Autodesk Inventor part; units mm, degrees
ref_plane "YZ Plane" through (0, 0, 0) normal (1, 0, 0) x (0, 1, 0)
ref_plane "XZ Plane" through (0, 0, 0) normal (0, 1, 0) x (-1, 0, 0)
ref_plane "XY Plane" through (0, 0, 0) normal (0, 0, 1) x (1, 0, 0)
sketch "Эскиз1" plane through (0, 0, 0) normal (0, 0, 1) x (1, 0, 0)
  arc A0 (-17.4305, 17.6734) -> (-22.4305, 12.6734) centre (-17.4305, 12.6734) ccw
  line L0 (-22.4305, 12.6734) -> (-22.4305, -4.8714)
  arc A1 (-22.4305, -4.8714) -> (-17.4305, -9.8714) centre (-17.4305, -4.8714) ccw
  line L1 (-17.4305, -9.8714) -> (-4.1609, -9.8714)
  line L2 (-4.1609, -9.8714) -> (-4.1609, -17.7214)
  arc A2 (-4.1609, -17.7214) -> (-0.1609, -21.7214) centre (-0.1609, -17.7214) ccw
  line L3 (-0.1609, -21.7214) -> (9.8391, -21.7214)
  arc A3 (9.8391, -21.7214) -> (14.8391, -16.7214) centre (9.8391, -16.7214) ccw
  line L4 (14.8391, -16.7214) -> (14.8391, -9.8714)
  line L5 (19.8391, -9.8714) -> (19.8391, 12.6734)
  arc A4 (19.8391, 12.6734) -> (14.8391, 17.6734) centre (14.8391, 12.6734) ccw
  line L6 (14.8391, 17.6734) -> (-17.4305, 17.6734)
  circle A5 centre (-11.2957, 3.901) radius 2.5
  circle A6 centre (4.8391, -17.7214) radius 1.5
  line L7 (14.8391, -9.8714) -> (19.8391, -9.8714)
  circle A7 centre (-11.2957, 13.465) radius 0.75
  circle A8 centre (-11.2957, -5.8075) radius 0.75
  point P0 (0, 0)
  dimension "d0" = 5
extrude "Выдавливание1" add sketch "Эскиз1" along normal blind 2
chamfer "Фаска3" distance 2 angle 45 1 edges at (-12.0457, -5.8075, 0)
chamfer "Фаска4" distance 2 angle 45 1 edges at (-12.0457, 13.465, 0)
properties part number "Верт держатели-2 правый"
Here's how the part is built. I have some questions about the finished solid (model axes, mm). A direction names the side the tool comes from. Give positions to 0.01 mm unless a question says otherwise; leave off trailing zeros. Order: outer loops, then holes, each group sorted by start corner. A loop starts at its lowest first (then second) coordinate and runs counter-clockwise, first axis right, second up. Notation, with made-up numbers: M 57.25,83 L 106.25,83 A11 ccw 106.25,92 Z; hole C -22.5,-4.75 d3. An arc over 180 degrees is marked long. Use a Markdown table: item, result. Add a question column.
1. On a 3-axis mill with a long thin cutter (end or side, diameter ignored), from which of +Z, -Z, +X, -X, +Y, -Y can I reach the whole of each face in a straight line? I mean faces 4 (the flat face through (-1, 17.673, 1)), 5 (the flat face through (-11, -9.871, 1)). Say none if no direction works.
2. Suppose I cut it at B-B (x = -15). List the corners of the cut face in (y, z) for me.
3. For pin 1 Ø1.7 at (x, y) = (-11.3, -5.81) entering from -Z; pin 2 Ø1 at (x, z) = (16.5, 1) entering from -Y; pin 3 Ø0.6 at (y, z) = (-13.5, 0.5) entering from +X, each with a flat end and sliding along its axis, tell me the tip position at first contact or that it passes through.
4. Suppose I cut it at A-A (z = 0.65). List the corners of the cut face in (x, y) for me (1 decimal), and give its area (3 significant figures).
5. Suppose I cut it at C-C (y = -14). List the corners of the cut face in (x, z) for me.
6. If we mould it in two halves opening along X, with no side actions, what happens to faces 1 (the flat face through (-22.43, 4, 1)), 2 (the cylindrical face through (18.336, 16.248, 0.986)), 3 (the cylindrical face through (-13.793, 3.791, 0.986))? For each: +X half, -X half, draft (parallel to the pull), parting line (faces both ways), or undercut.
7. I need wall thicknesses on probe 1 along Y at (x, z) = (5, 1.1); probe 2 along X at (y, z) = (-12.5, 1.7); probe 3 along Y at (x, z) = (-16.5, 0.45). Which ranges of each line are inside material? Lowest first, please. Write a range as from..to.
Results list:
| question | item | result |
|---|---|---|
| 1 | face 4 | +Z, -Z, +X, -X, +Y |
| 1 | face 5 | +Z, -Z, -X, -Y |
| 2 | outline | M -9.87,0 L 17.67,0 L 17.67,2 L -9.87,2 Z |
| 3 | pin 1 | stops at z = 1.89 |
| 3 | pin 2 | stops at y = -9.87 |
| 3 | pin 3 | stops at x = 14.84 |
| 4 | outline | M -22.4,-4.9 A5 ccw -17.4,-9.9 L -4.2,-9.9 L -4.2,-17.7 A4 ccw -0.2,-21.7 L 9.8,-21.7 A5 ccw 14.8,-16.7 L 14.8,-9.9 L 19.8,-9.9 L 19.8,12.7 A5 ccw 14.8,17.7 L -17.4,17.7 A5 ccw -22.4,12.7 Z; hole C -11.3,3.9 d5; hole C -11.3,-5.8 d4.2; hole C -11.3,13.5 d4.2; hole C 4.8,-17.7 d3 |
| 4 | area | 1,310 mm² |
| 5 | outline | M -4.16,0 L 14.84,0 L 14.84,2 L -4.16,2 Z |
| 6 | face 1 | -X half |
| 6 | face 2 | +X half |
| 6 | face 3 | undercut |
| 7 | probe 1 | y = -21.72..-19.21, -16.23..17.67 |
| 7 | probe 2 | x = -4.16..14.84 |
| 7 | probe 3 | y = -9.87..17.67 |
